from build123d import *

# Parameters (mm, degrees)
SKETCH003_W     = 40
SKETCH003_H     = 40
SKETCH003_R     = 2.05
PAD003_DEPTH    = 2
SKETCH006_W     = 32
SKETCH006_H     = 32
SKETCH006_W_2   = 14
SKETCH006_H_2   = 14
PAD005_DEPTH    = 10
SKETCH029_R     = 2
POCKET010_DEPTH = 8
SKETCH030_R     = 2
POCKET011_DEPTH = 8
SKETCH031_R     = 2
POCKET012_DEPTH = 8


with BuildPart() as part:
    # Sketch003 → Pad003 (new body)
    with BuildSketch(Plane.XZ):
        with Locations((0, 20)):
            Rectangle(SKETCH003_W, SKETCH003_H)
        with Locations((0, 20)):
            Circle(SKETCH003_R, mode=Mode.SUBTRACT)
    extrude(amount=PAD003_DEPTH)

    # Sketch006 (on Face6 of Pad003) → Pad005 (join)
    with BuildSketch(Plane(origin=(0, 0, 0), x_dir=(1, 0, 0), z_dir=(0, 1, 0))):
        with Locations((0, -20)):
            Rectangle(SKETCH006_W, SKETCH006_H)
        with Locations((0, -20)):
            Rectangle(SKETCH006_W_2, SKETCH006_H_2, mode=Mode.SUBTRACT)
    extrude(amount=PAD005_DEPTH)

    # Sketch029 (on Face8 of Pad005) → Pocket010 (cut)
    with BuildSketch(Plane(origin=(0, 0, 36), x_dir=(-1, 0, 0), z_dir=(0, 0, 1))):
        with Locations((-8, -5)):
            Circle(SKETCH029_R)
        with Locations((8, -5)):
            Circle(SKETCH029_R)
    extrude(amount=-POCKET010_DEPTH, mode=Mode.SUBTRACT)

    # Sketch030 (on Face7 of Pocket010) → Pocket011 (cut)
    with BuildSketch(Plane(origin=(-16, 0, 0), x_dir=(0, 0, -1), z_dir=(-1, 0, 0))):
        with Locations((-28, -5)):
            Circle(SKETCH030_R)
        with Locations((-12, -5)):
            Circle(SKETCH030_R)
    extrude(amount=-POCKET011_DEPTH, mode=Mode.SUBTRACT)

    # Sketch031 (on Face9 of Pocket011) → Pocket012 (cut)
    with BuildSketch(Plane(origin=(16, 0, 0), x_dir=(0, 0, 1), z_dir=(1, 0, 0))):
        with Locations((12, -5)):
            Circle(SKETCH031_R)
        with Locations((28, -5)):
            Circle(SKETCH031_R)
    extrude(amount=-POCKET012_DEPTH, mode=Mode.SUBTRACT)


with BuildPart() as part_1:
    # Body003 placement: moved
    add(part.part.moved(Location((0, -200, 0))))


solid = part_1.part
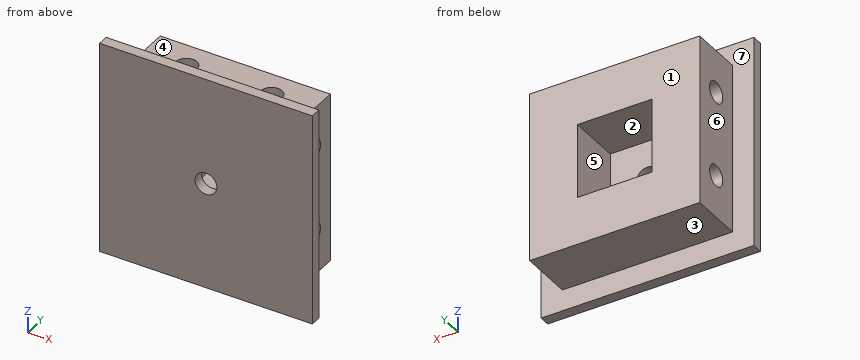
Model file for the job. Use its own axes, mm. Face numbers are marked on the shaded views. A direction names the side the tool comes from. Give positions to 0.01 mm unless a question says otherwise; leave off trailing zeros. Order: outer loops, then holes, each group sorted by start corner. A loop starts at its lowest first (then second) coordinate and runs counter-clockwise, first axis right, second up. Notation, with made-up numbers: M 67.5,62.5 L 99.5,62.5 A24 ccw 99.5,80.5 Z; hole C 38,8.5 d9. An arc over 180 degrees is marked long. Put each result on its own line as item: value. Start each with the question number.
(1) Band-saw the part on B-B on x = 0. Give the cut face in (y, z).
(2) Drill centre lines: L1, parallel to Z at x = -13, y = -195; L2, parallel to X at y = -195, z = 30.5; L3, parallel to Z at x = 2, y = -197.5. Where is each one in solid material? Low to high. Write a range as [from, to].
(3) Pull direction X, two halves, no side cores. Call the marked faces 5, 6 and 7: released by +X, released by -X, zero draft, split by the parting line, or undercut.
(4) Band-saw the part on A-A on y = -195. Count the separate pieces of the cut face and the enclosed holes in it, then the cut area to 3 significant figures.
(5) Band-saw the part on C-C on x = -4.5. Give the cut face in (y, z).
(6) Pin check, flat tips, straight feed: pin 1 Ø1.6 at (x, y) = (7, -194.5) entering from +Z; pin 2 Ø4.5 at (y, z) = (-195, 12) entering from +X; pin 3 Ø1.5 at (x, y) = (-15.5, -191.5) entering from -Z. Stop position of each tip, or through.
(7) Tool access for the marked faces 1, 2, 3 and 4: list every direction of +Z, -Z, +X, -X, +Y, -Y with a clear straight run to the whole face (end or side of a thin tool).
(8) Band-saw the part on D-D on y = -192. Give the cut face in (x, z).
Results below:
1. outline: M -202,0 L -200,0 L -200,4 L -190,4 L -190,13 L -200,13 L -200,17.95 L -202,17.95 Z; M -202,22.05 L -200,22.05 L -200,27 L -190,27 L -190,36 L -200,36 L -200,40 L -202,40 Z
2. L1: z = [4, 10], [14, 26], [30, 36]
2. L2: x = [-16, -10], [-6, 6], [10, 16]
2. L3: z = [4, 13], [27, 36]
3. face 5: undercut
3. face 6: released by -X
3. face 7: zero draft
4. separate pieces: 3
4. enclosed holes: 1
4. area: 644 mm2
5. outline: M -202,0 L -200,0 L -200,4 L -190,4 L -190,13 L -200,13 L -200,27 L -190,27 L -190,36 L -200,36 L -200,40 L -202,40 Z
6. pin 1: stops at z = 28
6. pin 2: stops at x = 16
6. pin 3: stops at z = 4
7. face 1: +Z, -Z, +X, -X, +Y
7. face 2: +Y
7. face 3: -Z, +X, -X, +Y
7. face 4: +Z, +X, -X, +Y
8. outline: M -16,4 L 16,4 L 16,36 L -16,36 Z; hole M -7,13 L 7,13 L 7,27 L -7,27 Z
